from build123d import *

# Parameters (mm, degrees)
BOSS_EXTRUDE1_DEPTH  = 12.5
SKETCH2_W            = 103
SKETCH2_H            = 83.5
CUT_EXTRUDE1_DEPTH   = 4
SKETCH3_W            = 103
SKETCH3_H            = 83.5
CUT_EXTRUDE2_DEPTH   = 6.5
SKETCH4_W            = 105
SKETCH4_H            = 85.5
SKETCH4_W_2          = 103
SKETCH4_H_2          = 83.5
BOSS_EXTRUDE2_DEPTH  = 1.5
SKETCH7_W            = 35
SKETCH7_H            = 4
CUT_EXTRUDE3_DEPTH   = 117.443387532
SKETCH8_W            = 7.5
SKETCH8_H            = 10
CUT_EXTRUDE4_DEPTH   = 2
SKETCH9_W            = 7.5
SKETCH9_H            = 10
CUT_EXTRUDE5_DEPTH   = 2
BOSS_EXTRUDE3_DEPTH  = 1.5
BOSS_EXTRUDE4_DEPTH  = 1.5
BOSS_EXTRUDE5_DEPTH  = 6
BOSS_EXTRUDE6_DEPTH  = 6
SKETCH14_W           = 28
SKETCH14_H           = 4
CUT_EXTRUDE6_DEPTH   = 2
SKETCH15_W           = 15
SKETCH15_H           = 3.5
CUT_EXTRUDE7_DEPTH   = 4
SKETCH16_R           = 1.25
SKETCH16_W           = 2
SKETCH16_H           = 24
CUT_EXTRUDE8_DEPTH   = 2
SKETCH17_R           = 2.5
SKETCH17_R_2         = 1.25
BOSS_EXTRUDE7_DEPTH  = 6.5
SKETCH18_W           = 28
SKETCH18_H           = 2
BOSS_EXTRUDE8_DEPTH  = 4
BOSS_EXTRUDE9_DEPTH  = 26
BOSS_EXTRUDE10_DEPTH = 26
BOSS_EXTRUDE11_DEPTH = 4
SKETCH22_W           = 22.25
SKETCH22_H           = 2
BOSS_EXTRUDE12_DEPTH = 2
SKETCH23_W           = 22.25
SKETCH23_H           = 2
BOSS_EXTRUDE13_DEPTH = 2


with BuildPart() as part:
    # Sketch1 → Boss-Extrude1 (new body)
    with BuildSketch(Plane(origin=(0, 0, 0), x_dir=(1, 0, 0), z_dir=(0, 1, 0))):
        with BuildLine():
            Line((52.5, -43.75), (-52.5, -43.75))
            ThreePointArc((-52.5, -43.75), (-53.207106781, -43.457106781), (-53.5, -42.75))
            Line((-53.5, -42.75), (-53.5, 42.75))
            ThreePointArc((-53.5, 42.75), (-53.207106781, 43.457106781), (-52.5, 43.75))
            Line((-52.5, 43.75), (52.5, 43.75))
            ThreePointArc((52.5, 43.75), (53.207106781, 43.457106781), (53.5, 42.75))
            Line((53.5, 42.75), (53.5, -42.75))
            ThreePointArc((53.5, -42.75), (53.207106781, -43.457106781), (52.5, -43.75))
        make_face()
    extrude(amount=BOSS_EXTRUDE1_DEPTH)

    # Sketch2 → Cut-Extrude1 (cut)
    with BuildSketch(Plane.XZ):
        Rectangle(SKETCH2_W, SKETCH2_H)
    extrude(amount=-CUT_EXTRUDE1_DEPTH, mode=Mode.SUBTRACT)

    # Sketch3 → Cut-Extrude2 (cut)
    with BuildSketch(Plane(origin=(0, 12.5, 0), x_dir=(1, 0, 0), z_dir=(0, 1, 0))):
        Rectangle(SKETCH3_W, SKETCH3_H)
    extrude(amount=-CUT_EXTRUDE2_DEPTH, mode=Mode.SUBTRACT)

    # Sketch4 → Boss-Extrude2 (add)
    with BuildSketch(Plane(origin=(0, 12.5, 0), x_dir=(1, 0, 0), z_dir=(0, 1, 0))):
        Rectangle(SKETCH4_W, SKETCH4_H)
        Rectangle(SKETCH4_W_2, SKETCH4_H_2, mode=Mode.SUBTRACT)
    extrude(amount=BOSS_EXTRUDE2_DEPTH)

    # Sketch7 → Cut-Extrude3 (cut, through all)
    with BuildSketch(Plane.ZY.offset(53.5)):
        with Locations((-0.25, 2)):
            Rectangle(SKETCH7_W, SKETCH7_H)
    extrude(amount=-CUT_EXTRUDE3_DEPTH, mode=Mode.SUBTRACT)

    # Sketch8 → Cut-Extrude4 (cut)
    with BuildSketch(Plane.ZY.offset(53.5)):
        with Locations((0, 9)):
            Rectangle(SKETCH8_W, SKETCH8_H)
    extrude(amount=-CUT_EXTRUDE4_DEPTH, mode=Mode.SUBTRACT)

    # Sketch9 → Cut-Extrude5 (cut)
    with BuildSketch(Plane(origin=(53.5, 0, 0), x_dir=(0, 0, -1), z_dir=(1, 0, 0))):
        with Locations((0, 9)):
            Rectangle(SKETCH9_W, SKETCH9_H)
    extrude(amount=-CUT_EXTRUDE5_DEPTH, mode=Mode.SUBTRACT)

    # Sketch10 → Boss-Extrude3 (add)
    with BuildSketch(Plane.ZY.offset(-51.5)):
        Polygon((5.5, 6), (-5.5, 6), (-5.5, 11), (-3, 11), (-3, 16.5), (3, 16.5), (3, 11), (5.5, 11), align=None)
    extrude(amount=BOSS_EXTRUDE3_DEPTH)

    # Sketch11 → Boss-Extrude4 (add)
    with BuildSketch(Plane(origin=(-51.5, 0, 0), x_dir=(0, 0, -1), z_dir=(1, 0, 0))):
        Polygon((-5.5, 11), (-5.5, 6), (5.5, 6), (5.5, 11), (3, 11), (3, 16.5), (-3, 16.5), (-3, 11), align=None)
    extrude(amount=BOSS_EXTRUDE4_DEPTH)

    # Sketch12 → Boss-Extrude5 (add)
    with BuildSketch(Plane(origin=(0, 0, -3), x_dir=(-1, 0, 0), z_dir=(0, 0, -1))):
        Polygon((-52.720588235, 16.5), (-50, 16.5), (-50, 19.5), (-51, 19.5), (-52.720588235, 17), align=None)
    extrude(amount=-BOSS_EXTRUDE5_DEPTH)

    # Sketch13 → Boss-Extrude6 (add)
    with BuildSketch(Plane(origin=(0, 0, -3), x_dir=(-1, 0, 0), z_dir=(0, 0, -1))):
        Polygon((50, 16.5), (52.5, 16.5), (52.5, 17), (51, 19.5), (50, 19.5), align=None)
    extrude(amount=-BOSS_EXTRUDE6_DEPTH)

    # Sketch14 → Cut-Extrude6 (cut)
    with BuildSketch(Plane.XZ.offset(-4)):
        with Locations((36.5, -15.75)):
            Rectangle(SKETCH14_W, SKETCH14_H)
        with Locations((-36.5, -15.75)):
            Rectangle(SKETCH14_W, SKETCH14_H)
    extrude(amount=-CUT_EXTRUDE6_DEPTH, mode=Mode.SUBTRACT)

    # Sketch15 → Cut-Extrude7 (cut)
    with BuildSketch(Plane.XZ):
        with Locations((0, 42)):
            Rectangle(SKETCH15_W, SKETCH15_H)
    extrude(amount=-CUT_EXTRUDE7_DEPTH, mode=Mode.SUBTRACT)

    # Sketch16 → Cut-Extrude8 (cut)
    with BuildSketch(Plane(origin=(0, 6, 0), x_dir=(1, 0, 0), z_dir=(0, 1, 0))):
        with Locations(Location((1.5, -23.5, 0), (0, 0, 270))):
            Circle(SKETCH16_R)
        with Locations((6.5, -28.75)):
            Rectangle(SKETCH16_W, SKETCH16_H)
        with Locations((-6.5, -28.75)):
            Rectangle(SKETCH16_W, SKETCH16_H)
    extrude(amount=-CUT_EXTRUDE8_DEPTH, mode=Mode.SUBTRACT)

    # Sketch17 → Boss-Extrude7 (add)
    # profile 1 of 4: a face of its own
    with BuildSketch(Plane(origin=(0, 6, 0), x_dir=(1, 0, 0), z_dir=(0, 1, 0))):
        with Locations(Location((42.5, 25, 0), (0, 0, 90))):
            Circle(SKETCH17_R)
        with Locations(Location((42.5, 25, 0), (0, 0, 90))):
            Circle(SKETCH17_R_2, mode=Mode.SUBTRACT)
    # profile 2 of 4: a face of its own
    with BuildSketch(Plane(origin=(0, 6, 0), x_dir=(1, 0, 0), z_dir=(0, 1, 0))):
        with Locations(Location((42.5, -25, 0), (0, 0, 90))):
            Circle(SKETCH17_R)
        with Locations(Location((42.5, -25, 0), (0, 0, 90))):
            Circle(SKETCH17_R_2, mode=Mode.SUBTRACT)
    # profile 3 of 4: a face of its own
    with BuildSketch(Plane(origin=(0, 6, 0), x_dir=(1, 0, 0), z_dir=(0, 1, 0))):
        with Locations(Location((-42.5, 25, 0), (0, 0, 90))):
            Circle(SKETCH17_R)
        with Locations(Location((-42.5, 25, 0), (0, 0, 90))):
            Circle(SKETCH17_R_2, mode=Mode.SUBTRACT)
    # profile 4 of 4: a face of its own
    with BuildSketch(Plane(origin=(0, 6, 0), x_dir=(1, 0, 0), z_dir=(0, 1, 0))):
        with Locations(Location((-42.5, -25, 0), (0, 0, 90))):
            Circle(SKETCH17_R)
        with Locations(Location((-42.5, -25, 0), (0, 0, 90))):
            Circle(SKETCH17_R_2, mode=Mode.SUBTRACT)
    extrude(amount=BOSS_EXTRUDE7_DEPTH)

    # Sketch18 → Boss-Extrude8 (add)
    with BuildSketch(Plane.XZ.offset(-4)):
        with Locations((-37.5, -18.75)):
            Rectangle(SKETCH18_W, SKETCH18_H)
        with Locations((37.5, -18.75)):
            Rectangle(SKETCH18_W, SKETCH18_H)
    extrude(amount=BOSS_EXTRUDE8_DEPTH)

    # Sketch19 → Boss-Extrude9 (add)
    with BuildSketch(Plane.ZY.offset(-23.5)):
        Polygon((-17.75, 0), (-14.75, 0), (-14.75, 1), (-15.75, 2), (-17.75, 2), align=None)
    extrude(amount=-BOSS_EXTRUDE9_DEPTH)

    # Sketch20 → Boss-Extrude10 (add)
    with BuildSketch(Plane(origin=(-23.5, 0, 0), x_dir=(0, 0, -1), z_dir=(1, 0, 0))):
        Polygon((14.75, 0), (17.75, 0), (17.75, 2), (15.75, 2), (14.75, 1), align=None)
    extrude(amount=-BOSS_EXTRUDE10_DEPTH)

    # Sketch21 → Boss-Extrude11 (add)
    with BuildSketch(Plane.XZ.offset(-4)):
        Polygon((7.5, 41.75), (7.5, 17.75), (40.5, 17.75), (43.496447897, 19.48), (42.497454433, 21.215), (39.96, 19.75), (9.5, 19.75), (9.5, 41.75), align=None)
        Polygon((-7.5, 41.75), (-7.5, 17.75), (-40.5, 17.75), (-43.496447897, 19.48), (-42.497454433, 21.215), (-39.96, 19.75), (-9.5, 19.75), (-9.5, 41.75), align=None)
    extrude(amount=BOSS_EXTRUDE11_DEPTH)

    # Sketch22 → Boss-Extrude12 (add)
    with BuildSketch(Plane.ZY.offset(-7.5)):
        with Locations((29.125, 1)):
            Rectangle(SKETCH22_W, SKETCH22_H)
    extrude(amount=BOSS_EXTRUDE12_DEPTH)

    # Sketch23 → Boss-Extrude13 (add)
    with BuildSketch(Plane(origin=(-7.5, 0, 0), x_dir=(0, 0, -1), z_dir=(1, 0, 0))):
        with Locations((-29.125, 1)):
            Rectangle(SKETCH23_W, SKETCH23_H)
    extrude(amount=BOSS_EXTRUDE13_DEPTH)


solid = part.part
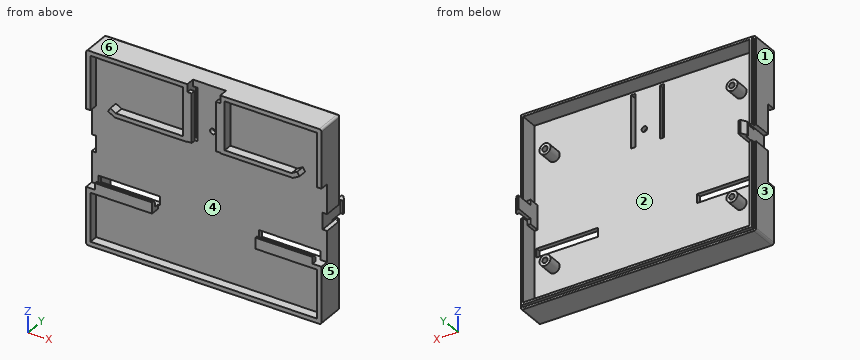
Design review of the part built by this model. Coordinates are the model's own, in mm. Face numbers are marked on the shaded views. A direction names the side the tool comes from. Give positions to 0.01 mm unless a question says otherwise; leave off trailing zeros. Loops run counter-clockwise (first coordinate to the right, second up) from the corner with the lowest first, then second, coordinate; pieces in that order, holes last. Notation, with made-up numbers: (82.5, -1) - (130.5, -1) arc R20 cw to (130.5, 27) - close; hole circle Ø7 at (18, 87). An arc over 180 degrees is marked (long way). Use CSV: the item, a comma, the result in double quotes. Start each with the question number.
1. Add section C-C (x = 1.5). State the section outline as (y, z) points, plus the area to 3 significant figures.
2. Insertion check: P1, Ø6, axis at x = 24.5, y = 13.5, coming from the +Z side; P2, Ø3, axis at x = 8.5, z = 11.5, coming from the -Y side; P3, Ø5, axis at y = 17.5, z = 8.5, coming from the -X side; P4, Ø2.5, axis at x = 42, z = 25.5, coming from the +Y side. Each pin has a flat end and moves straight along its axis. Give the tip position at first contact, or say it passes through.
3. Wall thickness on L1, parallel to Z at x = -42.5, y = 7.5; L2, parallel to X at y = 11, z = -25; L3, parallel to Z at x = 44.5, y = 11.75: over which ranges is each line inside the solid? List them lowest first.
4. Draft analysis for pull direction X (two halves, no side actions). For the marked faces 3, 4, 5 and 6, state which applies: released by +X, released by -X, zero draft, split by the parting line, or undercut.
5. Machinability: for the marked faces 1 and 2, which of the approach directions +Z, -Z, +X, -X, +Y, -Y give a long, thin tool a straight path to every point of the face, cutting with its end or side? Answer none if there is none.
6. Add section B-B (z = 32.5). Count the separate pieces of the cut face and the enclosed holes in it, plus the area to 3 significant figures.
Results found:
1,outline,"(0, -43.75) - (12.5, -43.75) - (12.5, -42.75) - (14, -42.75) - (14, -41.75) - (6, -41.75) - (6, 22.25) - (4, 22.25) - (4, -41.75) - (0, -41.75) - close; (4, 24.75) - (6, 24.75) - (6, 41.75) - (14, 41.75) - (14, 42.75) - (12.5, 42.75) - (12.5, 43.75) - (4, 43.75) - close"
1,area,"207 mm²"
2,P1,"stops at z = 43.75"
2,P2,"stops at y = 4"
2,P3,"passes through"
2,P4,"stops at y = 12.5"
3,L1,"z = -43.75 to -41.75, -27.5 to -26.25, -23.75 to -22.5, 22.5 to 23.75, 26.25 to 27.5, 41.75 to 43.75"
3,L2,"x = -53.5 to -51.5, -45 to -43.75, -41.25 to -40, 40 to 41.25, 43.75 to 45, 51.5 to 53.5"
3,L3,"z = -43.75 to -41.75, -26.5 to -23.5, 23.5 to 26.5, 41.75 to 43.75"
4,face 3,"released by -X"
4,face 4,"undercut"
4,face 5,"released by +X"
4,face 6,"zero draft"
5,face 1,"+Z, -Z, -X, +Y, -Y"
5,face 2,"+Y"
6,separate pieces,"3"
6,enclosed holes,"0"
6,area,"275 mm²"
